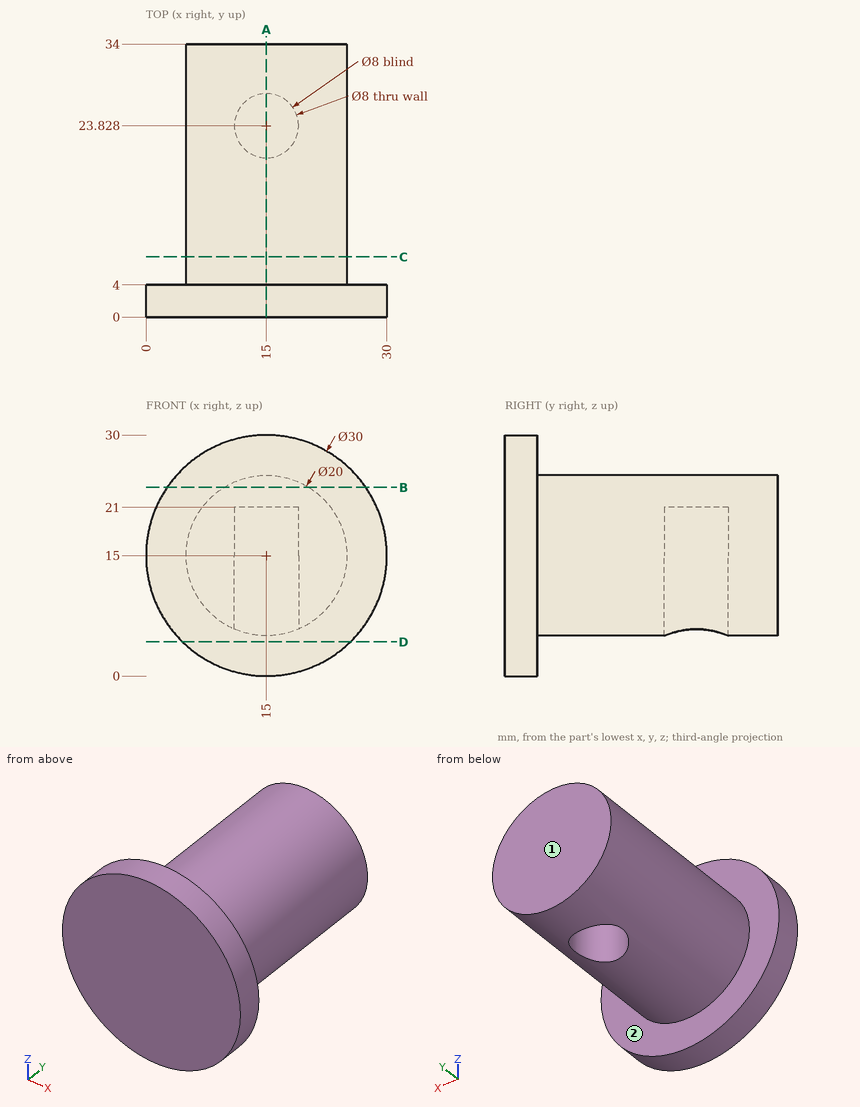
Input: dimensioned drawing with shaded views. Units: mm. Origin: part minimum x, y, z. A direction names the side the tool comes from. Give positions to 0.01 mm unless a question says otherwise; leave off trailing zeros. Loops run counter-clockwise (first coordinate to the right, second up) from the corner with the lowest first, then second, coordinate; pieces in that order, holes last. Notation, with made-up numbers: (14.25, -23.75) -> (43.25, -23.75) arc R24 cw to (43.25, 13.25) -> close; hole circle Ø4 at (77.25, 58.5). An arc over 180 degrees is marked (long way). Use a Markdown table: item, result.
Q1. Access query for the marked faces 1 and 2. Directions: +Z, -Z, +X, -X, +Y, -Y. A direction counts if a zero-diameter tool reaches every point of the face in a straight line with its end or side. Return the directions, or none.
Entries:
| item | result |
|---|---|
| face 1 | +Z, -Z, +X, -X, +Y |
| face 2 | +Y |
Q2. Ray query, probe 1 along Y at (x, z) = (15, 11.5); probe 2 along Y at (x, z) = (7.25, 7); probe 3 along X at (y, z) = (26, 12). Return the intervals inside material, ascending. Write a range as from..to.
Entries:
| item | result |
|---|---|
| probe 1 | y = 0..19.83, 27.83..34 |
| probe 2 | y = 0..4 |
| probe 3 | x = 5.46..11.64, 18.36..24.54 |
Q3. Section query D-D, the plane z = 4.25. Return the cut outline in (x, y), plus the area to 3 significant figures.
Entries:
| item | result |
|---|---|
| outline | (4.54, 0) -> (25.46, 0) -> (25.46, 4) -> (4.54, 4) -> close |
| area | 83.7 mm² |
Q4. Section query C-C, the plane y = 7.5. Return the cut outline in (x, z), plus the area to 3 significant figures.
Entries:
| item | result |
|---|---|
| outline | circle Ø20 at (15, 15) |
| area | 314 mm² |
Q5. Section query A-A, the plane x = 15. Return the cut outline in (y, z).
Entries:
| item | result |
|---|---|
| outline | (0, 0) -> (4, 0) -> (4, 5) -> (19.83, 5) -> (19.83, 21) -> (27.83, 21) -> (27.83, 5) -> (34, 5) -> (34, 25) -> (4, 25) -> (4, 30) -> (0, 30) -> close |
Q6. Section query B-B, the plane z = 23.5. Return the cut outline in (x, y), plus the area to 3 significant figures.
Entries:
| item | result |
|---|---|
| outline | (2.64, 0) -> (27.36, 0) -> (27.36, 4) -> (20.27, 4) -> (20.27, 34) -> (9.73, 34) -> (9.73, 4) -> (2.64, 4) -> close |
| area | 415 mm² |
Q7. First-contact query: P1, Ø6.5, axis at x = 15.5, y = 23.5, coming from the -Z side; P2, Ø10, axis at y = 16, z = 8, coming from the +X side; P3, Ø2, axis at y = 17, z = 10.5, coming from the -X side; P4, Ø10, axis at x = 9.5, z = 25.5, coming from the -Y side. Flat tips, straight axial feed; report the tip coordinate or a pass-through.
Entries:
| item | result |
|---|---|
| P1 | stops at z = 21 |
| P2 | stops at x = 24.8 |
| P3 | stops at x = 5.63 |
| P4 | stops at y = 0 |
